The model under review builds one solid part; all positions refer to its coordinate system, in mm. A direction names the side the tool comes from. Round coordinates to 2 decimals unless told otherwise and drop trailing zeros. Order: outer loops, then holes, each group sorted by start corner. A loop starts at its lowest first (then second) coordinate and runs counter-clockwise, first axis right, second up. Notation, with made-up numbers: (63, 70.5) -> (97, 70.5) arc R10 ccw to (97, 83.5) -> close; hole circle Ø3 at (26, -35). An arc over 180 degrees is marked (long way). Use a Markdown table: item, result. Add a question column.
```python
from build123d import *

# Parameters (mm, degrees)
SKETCH_1_W          = 130
SKETCH_1_H          = 90
SKETCH_1_R          = 1.5
EXTRUDE_1_DEPTH     = 2
CUT_EXTRUDE_1_DEPTH = 3
CUT_EXTRUDE_2_DEPTH = 3
CUT_EXTRUDE_3_DEPTH = 3
SKETCH_6_R          = 0.75
SKETCH_6_R_2        = 0.5
CUT_EXTRUDE_5_DEPTH = 10
CUT_EXTRUDE_7_DEPTH = 3


with BuildPart() as part:
    # 草图1 → 凸台-拉伸1 (new body)
    with BuildSketch(Plane.XY):
        with Locations((65, 45)):
            Rectangle(SKETCH_1_W, SKETCH_1_H)
        with Locations((10, 10)):
            Circle(SKETCH_1_R, mode=Mode.SUBTRACT)
        with Locations((10, 30)):
            Circle(SKETCH_1_R, mode=Mode.SUBTRACT)
        with Locations((10, 50)):
            Circle(SKETCH_1_R, mode=Mode.SUBTRACT)
        with Locations((40, 10)):
            Circle(SKETCH_1_R, mode=Mode.SUBTRACT)
        with Locations((70, 10)):
            Circle(SKETCH_1_R, mode=Mode.SUBTRACT)
        with Locations((100, 10)):
            Circle(SKETCH_1_R, mode=Mode.SUBTRACT)
    extrude(amount=EXTRUDE_1_DEPTH)

    # 草图2 → 切除-拉伸1 (cut, through all)
    with BuildSketch(Plane.XY.offset(2)):
        Polygon((27, 90), (130, 46.702786812), (130, 90), align=None)
    extrude(amount=-CUT_EXTRUDE_1_DEPTH, mode=Mode.SUBTRACT)

    # 草图3 → 切除-拉伸2 (cut, through all)
    with BuildSketch(Plane.XY.offset(2)):
        Polygon((35.084739839, 86.601488307), (106.068202512, 56.76278815), (100.642984301, 43.856704028), (29.659521629, 73.695404185), align=None)
    extrude(amount=-CUT_EXTRUDE_2_DEPTH, mode=Mode.SUBTRACT)

    # 草图4 → 切除-拉伸3 (cut, through all)
    with BuildSketch(Plane.XY.offset(2)):
        Polygon((30.769088039, 84.07658246), (26.893932174, 74.857950944), (25.04098724, 75.636857273), (28.916143104, 84.855488789), align=None)
        Polygon((107.283729621, 51.912788784), (103.408573756, 42.694157268), (105.252300059, 41.919126096), (109.127455924, 51.137757611), align=None)
        Polygon((26.653248567, 71.704845903), (34.950016931, 68.217205625), (33.787470172, 65.45161617), (25.490701807, 68.939256448), align=None)
        Polygon((41.403058992, 65.504596519), (47.856101053, 62.791987414), (46.693554294, 60.02639796), (40.240512233, 62.739007065), align=None)
        Polygon((80.121311359, 49.228941888), (86.57435342, 46.516332783), (85.41180666, 43.750743329), (78.958764599, 46.463352434), align=None)
        Polygon((93.027395481, 43.803723678), (101.324163845, 40.3160834), (100.161617086, 37.550493945), (91.864848722, 41.038134223), align=None)
        Polygon((54.309143114, 60.079378309), (60.762185175, 57.366769204), (59.599638416, 54.601179749), (53.146596355, 57.313788854), align=None)
        Polygon((67.215227236, 54.654160099), (73.668269298, 51.941550994), (72.505722538, 49.175961539), (66.052680477, 51.888570644), align=None)
    extrude(amount=-CUT_EXTRUDE_3_DEPTH, mode=Mode.SUBTRACT)

    # 草图6 → 切除-拉伸5 (cut)
    with BuildSketch(Plane.XY.offset(2)):
        with Locations((25.490701807, 68.939256448)):
            Circle(SKETCH_6_R)
        with Locations((26.653248567, 71.704845903)):
            Circle(SKETCH_6_R)
        with Locations((34.950016931, 68.217205625)):
            Circle(SKETCH_6_R)
        with Locations((33.787470172, 65.45161617)):
            Circle(SKETCH_6_R)
        with Locations((46.693554294, 60.02639796)):
            Circle(SKETCH_6_R)
        with Locations((40.240512233, 62.739007065)):
            Circle(SKETCH_6_R)
        with Locations((41.403058992, 65.504596519)):
            Circle(SKETCH_6_R)
        with Locations((47.856101053, 62.791987414)):
            Circle(SKETCH_6_R)
        with Locations((80.121311359, 49.228941888)):
            Circle(SKETCH_6_R)
        with Locations((78.958764599, 46.463352434)):
            Circle(SKETCH_6_R)
        with Locations((85.41180666, 43.750743329)):
            Circle(SKETCH_6_R)
        with Locations((86.57435342, 46.516332783)):
            Circle(SKETCH_6_R)
        with Locations((100.161617086, 37.550493945)):
            Circle(SKETCH_6_R)
        with Locations((101.324163845, 40.3160834)):
            Circle(SKETCH_6_R)
        with Locations((93.027395481, 43.803723678)):
            Circle(SKETCH_6_R)
        with Locations((91.864848722, 41.038134223)):
            Circle(SKETCH_6_R)
        with Locations((26.893932174, 74.857950944)):
            Circle(SKETCH_6_R_2)
        with Locations((25.04098724, 75.636857273)):
            Circle(SKETCH_6_R_2)
        with Locations((28.916143104, 84.855488789)):
            Circle(SKETCH_6_R_2)
        with Locations((30.769088039, 84.07658246)):
            Circle(SKETCH_6_R_2)
        with Locations((105.252300059, 41.919126096)):
            Circle(SKETCH_6_R_2)
        with Locations((103.408573756, 42.694157268)):
            Circle(SKETCH_6_R_2)
        with Locations((107.283729621, 51.912788784)):
            Circle(SKETCH_6_R_2)
        with Locations((109.127455924, 51.137757611)):
            Circle(SKETCH_6_R_2)
        with Locations((54.309143114, 60.079378309)):
            Circle(SKETCH_6_R)
        with Locations((60.762185175, 57.366769204)):
            Circle(SKETCH_6_R)
        with Locations((53.146596355, 57.313788854)):
            Circle(SKETCH_6_R)
        with Locations((59.599638416, 54.601179749)):
            Circle(SKETCH_6_R)
        with Locations((67.215227236, 54.654160099)):
            Circle(SKETCH_6_R)
        with Locations((73.668269298, 51.941550994)):
            Circle(SKETCH_6_R)
        with Locations((72.505722538, 49.175961539)):
            Circle(SKETCH_6_R)
        with Locations((66.052680477, 51.888570644)):
            Circle(SKETCH_6_R)
    extrude(amount=-CUT_EXTRUDE_5_DEPTH, mode=Mode.SUBTRACT)

    # 草图8 → 切除-拉伸7 (cut, through all)
    with BuildSketch(Plane(origin=(0, 0, 0), x_dir=(-1, 0, 0), z_dir=(0, 0, -1))):
        with BuildLine():
            Line((-90, 14), (-80, 14))
            ThreePointArc((-80, 14), (-78.585786438, 13.414213562), (-78, 12))
            Line((-78, 12), (-78, 8))
            ThreePointArc((-78, 8), (-78.585786438, 6.585786438), (-80, 6))
            Line((-80, 6), (-90, 6))
            ThreePointArc((-90, 6), (-91.414213562, 6.585786438), (-92, 8))
            Line((-92, 8), (-92, 12))
            ThreePointArc((-92, 12), (-91.414213562, 13.414213562), (-90, 14))
        make_face()
        with BuildLine():
            Line((-62, 8), (-62, 12))
            ThreePointArc((-62, 12), (-61.414213562, 13.414213562), (-60, 14))
            Line((-60, 14), (-50, 14))
            ThreePointArc((-50, 14), (-48.585786438, 13.414213562), (-48, 12))
            Line((-48, 12), (-48, 8))
            ThreePointArc((-48, 8), (-48.585786438, 6.585786438), (-50, 6))
            Line((-50, 6), (-60, 6))
            ThreePointArc((-60, 6), (-61.414213562, 6.585786438), (-62, 8))
        make_face()
        with BuildLine():
            Line((-30, 14), (-20, 14))
            ThreePointArc((-20, 14), (-18.585786438, 13.414213562), (-18, 12))
            Line((-18, 12), (-18, 8))
            ThreePointArc((-18, 8), (-18.585786438, 6.585786438), (-20, 6))
            Line((-20, 6), (-30, 6))
            ThreePointArc((-30, 6), (-31.414213562, 6.585786438), (-32, 8))
            Line((-32, 8), (-32, 12))
            ThreePointArc((-32, 12), (-31.414213562, 13.414213562), (-30, 14))
        make_face()
    extrude(amount=-CUT_EXTRUDE_7_DEPTH, mode=Mode.SUBTRACT)


solid = part.part
```
Q1. To check wall thickness, follow line 1 along Y through (x, z) = (70, 1.4); line 2 along Y through (x, z) = (100, 1.3); line 3 along X through (y, z) = (60.5, 0.9). State the ranges of each line that lie inside material, in increasing order.
Q2. For faces 1 (the face through (30.986, 88.325, 1.014)), 2 (the face through (103.394, 50.4, 1.014)), 3 (the face through (28.86, 79.53, 1.01)), list the 3-axis set-ups (+Z, -Z, +X, -X, +Y, -Y) from which the entire face can be reached by the end or side of a thin tool; tool diameter is ignored.
Q3. Add section A-A, the plane y = 30. Give the boundary of the cut face in (x, z), then the cut area to 3 significant figures.
Q4. Add section D-D, the plane z = 1.05. Give the number of separate pieces and of enclosed holes in the cut face, then the cut area to 3 significant figures.
Q5. Draft analysis for pull direction X (two halves, no side actions). For faces 4 (the face through (32.334, 80.058, 1.014)), 5 (the face through (96.062, 39.274, 1.014)), 6 (the face through (50, 36, 2)), 7 (the face through (107.165, 46.47, 1.014)), state which applies: released by +X, released by -X, zero draft, split by the parting line, or undercut.
Q6. Add section B-B, the plane x = 10. Give the boundary of the cut face in (y, z), then the cut area to 3 significant figures.
Q7. Add section C-C, the plane x = 70. Give the boundary of the cut face in (y, z).
Q8. For pin 1 (1.2 mm diameter, centred on x = 60.76, y = 57.37, fed in from +Z), flat-tipped, find the tip position at first contact; note if it passes through.
Return value:
| question | item | result |
|---|---|---|
| 1 | line 1 | 0 to 8.5, 11.5 to 50.23, 53.48 to 56.74 |
| 1 | line 2 | 0 to 8.5, 11.5 to 36.82, 40.87 to 44.13 |
| 1 | line 3 | 0 to 45.57, 47.28 to 53.69, 54.93 to 61.05 |
| 2 | face 1 | +Z, -Z, +X, +Y |
| 2 | face 2 | +Z, -Z, +Y |
| 2 | face 3 | +Z, -Z |
| 3 | outline | (0, 0) -> (8.5, 0) -> (8.5, 2) -> (0, 2) -> close; (11.5, 0) -> (130, 0) -> (130, 2) -> (11.5, 2) -> close |
| 3 | area | 254 mm² |
| 4 | separate pieces | 1 |
| 4 | enclosed holes | 17 |
| 4 | area | 7,810 mm² |
| 5 | face 4 | released by +X |
| 5 | face 5 | undercut |
| 5 | face 6 | zero draft |
| 5 | face 7 | undercut |
| 6 | outline | (0, 0) -> (8.5, 0) -> (8.5, 2) -> (0, 2) -> close; (11.5, 0) -> (28.5, 0) -> (28.5, 2) -> (11.5, 2) -> close; (31.5, 0) -> (48.5, 0) -> (48.5, 2) -> (31.5, 2) -> close; (51.5, 0) -> (90, 0) -> (90, 2) -> (51.5, 2) -> close |
| 6 | area | 162 mm² |
| 7 | outline | (0, 0) -> (8.5, 0) -> (8.5, 2) -> (0, 2) -> close; (11.5, 0) -> (50.23, 0) -> (50.23, 2) -> (11.5, 2) -> close; (53.48, 0) -> (56.74, 0) -> (56.74, 2) -> (53.48, 2) -> close |
| 8 | pin 1 | through |
